Geometry: final body of the model. Coordinates: model frame, mm. Face numbers are marked on the shaded views. A direction names the side the tool comes from. Give positions to 0.01 mm unless a question says otherwise; leave off trailing zeros. Write each loop counter-clockwise with the first axis right and the second up, starting at its lowest first coordinate (ties: lowest second). Pieces come first, ordered by that corner, then holes.
Q1. Cut plane A-A on x = -7.5. Return the cut outline in (y, z) (3 decimals).
Q2. Cut plane C-C on z = -0.5. Return the cut outline in (x, y) (3 decimals).
Q3. Pin query (flat end, axial travel): pin 1 (3 mm diameter, centred on y = -1, z = -4.5, fed in from -X); pin 2 (6 mm diameter, centred on y = -5, z = 3, fed in from -X); pin 3 (2 mm diameter, centred on y = -6.5, z = 7, fed in from +X). Return the tip coordinate at first contact, or that it passes through.
Q4. Line query: L1, parallel to Y at x = 13.25, z = 6.35; L2, parallel to Z at x = 14, y = -19; L3, parallel to Y at x = -13, z = -10.75 (3 decimals). Output: solid intervals per line, ascending.
Q5. Cut plane D-D on x = 14. Return the cut outline in (y, z).
Q6. Cut plane B-B on y = 4.5. Return the cut outline in (x, z), plus the area to 3 significant figures.
Q7. Draft query along X for the marked faces 4, 5 and 6. Return one class per face: pulls with the +X half, pulls with the -X half, needs draft (parallel to the pull), parting line crosses it, or undercut.
Q8. Reachability of the marked faces 1, 2 and 3 from +Z, -Z, +X, -X, +Y, -Y: full face, straight path, thin tool, end or side. Return the list, or none.
```python
from build123d import *

# Parameters (mm, degrees)
SKETCH1_W                      = 38.1
SKETCH1_H                      = 25.4
BOSS_EXTRUDE1_DEPTH            = 12.7
CUT_EXTRUDE2_REACH             = 36.196
SKETCH7_R                      = 3.175
F_6_32_TAPPED_HOLE1_AT_2_COUNT = 2
F_6_32_TAPPED_HOLE1_AT_2_PITCH = 12.7
CUT_EXTRUDE3_DEPTH             = 25.4
SKETCH14_W                     = 28.575
SKETCH14_H                     = 12.7
CUT_EXTRUDE5_DEPTH             = 25.4
FILLET2_R                      = 3.175
FILLET2_OF_MIRROR1_R           = 3.175
FILLET3_R                      = 3.175


with BuildPart() as part:
    # Sketch1 → Boss-Extrude1 (new, symmetric)
    with BuildSketch(Plane.XY):
        Rectangle(SKETCH1_W, SKETCH1_H)
    boss_extrude1 = extrude(amount=BOSS_EXTRUDE1_DEPTH, both=True)

    # Sketch7 → Cut-Extrude2 (cut, up to next)
    with BuildSketch(Plane.XY.offset(12.7), mode=Mode.PRIVATE) as cut_extrude2_sk1:
        with Locations((19.05, -6.35)):
            Circle(SKETCH7_R)
    cut_extrude2_tool1 = extrude(cut_extrude2_sk1.sketch, amount=-CUT_EXTRUDE2_REACH, mode=Mode.PRIVATE) & part.part
    cut_extrude2 = cut_extrude2_tool1.solids().sort_by_distance((19.05, -6.35, 12.7))[0]
    add(cut_extrude2, mode=Mode.SUBTRACT)

    # Sketch11 → #6-32 Tapped Hole1 (revolve, cut)
    with BuildSketch(Plane(origin=(19.05, 6.35, 6.35), x_dir=(0, 0, -1), z_dir=(0, 1, 0))):
        Polygon((0, 0), (0, 8.89), (1.35255, 8.07730597), (1.35255, 0), align=None)
    f_6_32_tapped_hole1 = revolve(axis=Axis((25.4, 6.35, 6.35), (-1, 0, 0)), mode=Mode.SUBTRACT)

    # #6-32 Tapped Hole1 at 2: #6-32 Tapped Hole1 ×2
    with Locations(*[(0, 0, -i * F_6_32_TAPPED_HOLE1_AT_2_PITCH) for i in range(1, F_6_32_TAPPED_HOLE1_AT_2_COUNT)]):
        add(f_6_32_tapped_hole1, mode=Mode.SUBTRACT)

    # Sketch12 → Cut-Extrude3 (cut)
    with BuildSketch(Plane.XY.offset(12.7)):
        with BuildLine():
            Line((-13.335, 9.525), (5.715, 9.525))
            ThreePointArc((5.715, 9.525), (8.89, 6.35), (5.715, 3.175))
            Line((5.715, 3.175), (-13.335, 3.175))
            ThreePointArc((-13.335, 3.175), (-16.51, 6.35), (-13.335, 9.525))
        make_face()
    cut_extrude3 = extrude(amount=-CUT_EXTRUDE3_DEPTH, mode=Mode.SUBTRACT)

    # Sketch14 → Cut-Extrude5 (cut)
    with BuildSketch(Plane.XY.offset(12.7)):
        with Locations((-4.7625, -6.35)):
            Rectangle(SKETCH14_W, SKETCH14_H)
    cut_extrude5 = extrude(amount=-CUT_EXTRUDE5_DEPTH, mode=Mode.SUBTRACT)

    # Fillet2
    fillet2_edges = [part.edges().sort_by_distance(p)[0] for p in [
        (-19.05, 0, 0),
        (9.525, 0, 0),
        (-19.05, 12.7, 0),
    ]]
    fillet(fillet2_edges, radius=FILLET2_R)

    # Mirror1: Boss-Extrude1, Cut-Extrude2, #6-32 Tapped Hole1, Cut-Extrude3, Cut-Extrude5 across plane
    add(boss_extrude1.mirror(Plane.ZX.offset(-6.35)))
    add(cut_extrude2.mirror(Plane.ZX.offset(-6.35)), mode=Mode.SUBTRACT)
    add(f_6_32_tapped_hole1.mirror(Plane.ZX.offset(-6.35)), mode=Mode.SUBTRACT)
    add(cut_extrude3.mirror(Plane.ZX.offset(-6.35)), mode=Mode.SUBTRACT)
    add(cut_extrude5.mirror(Plane.ZX.offset(-6.35)), mode=Mode.SUBTRACT)

    # Mirror1 copy 1 sketch → Mirror1 copy 1 (revolve, cut)
    with BuildSketch(Plane(origin=(19.05, -19.05, -6.35), x_dir=(0, 0, -1), z_dir=(0, -1, 0))):
        Polygon((0, 0), (0, -8.89), (1.35255, -8.07730597), (1.35255, 0), align=None)
    revolve(axis=Axis((25.4, -19.05, -6.35), (1, 0, 0)), mode=Mode.SUBTRACT)

    # Fillet2 of Mirror1
    fillet2_of_mirror1_edges = [part.edges().sort_by_distance(p)[0] for p in [
        (-19.05, -12.7, 0),
        (9.525, -12.7, 0),
        (-19.05, -25.4, 0),
    ]]
    fillet(fillet2_of_mirror1_edges, radius=FILLET2_OF_MIRROR1_R)

    # Fillet3
    fillet3_edges = [part.edges().sort_by_distance(p)[0] for p in [
        (9.525, 0, 0),
    ]]
    fillet(fillet3_edges, radius=FILLET3_R)


solid = part.part
```
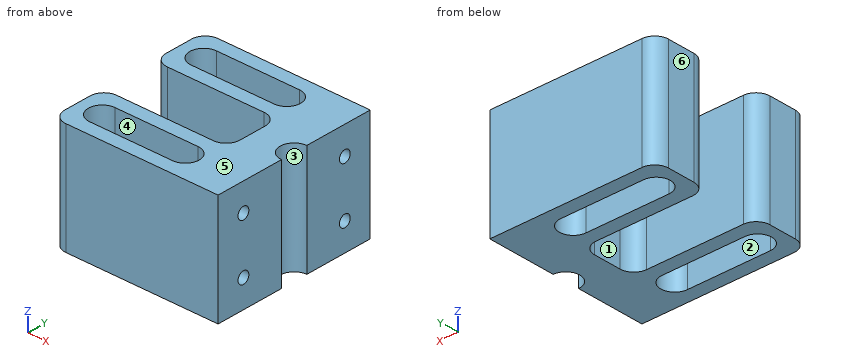
Data:
1. outline: (-25.4, -12.7) - (-22.225, -12.7) - (-22.225, 12.7) - (-25.4, 12.7) - close; (-15.875, -12.7) - (-12.7, -12.7) - (-12.7, 12.7) - (-15.875, 12.7) - close; (0, -12.7) - (3.175, -12.7) - (3.175, 12.7) - (0, 12.7) - close; (9.525, -12.7) - (12.7, -12.7) - (12.7, 12.7) - (9.525, 12.7) - close
2. outline: (-19.05, -22.225) arc R3.175 ccw to (-15.875, -25.4) - (19.05, -25.4) - (19.05, -9.525) arc R3.175 cw to (19.05, -3.175) - (19.05, 12.7) - (-15.875, 12.7) arc R3.175 ccw to (-19.05, 9.525) - (-19.05, 3.175) arc R3.175 ccw to (-15.875, 0) - (6.35, 0) arc R3.175 cw to (9.525, -3.175) - (9.525, -9.525) arc R3.175 cw to (6.35, -12.7) - (-15.875, -12.7) arc R3.175 ccw to (-19.05, -15.875) - close; hole (-13.335, -22.225) - (5.715, -22.225) arc R3.175 ccw to (5.715, -15.875) - (-13.335, -15.875) arc R3.175 ccw to start; hole (-13.335, 3.175) - (5.715, 3.175) arc R3.175 ccw to (5.715, 9.525) - (-13.335, 9.525) arc R3.175 ccw to start
3. pin 1: stops at x = -17.59
3. pin 2: stops at x = 9.3
3. pin 3: stops at x = 16.09
4. L1: y = -25.4 to -20.4, -17.7 to 5, 7.7 to 12.7
4. L2: z = -12.7 to -7.7, -5 to 5, 7.7 to 12.7
4. L3: y = -25.4 to -22.225, -15.875 to -12.7, 0 to 3.175, 9.525 to 12.7
5. outline: (-25.4, -12.7) - (12.7, -12.7) - (12.7, 12.7) - (-25.4, 12.7) - close; hole circle Ø2.71 at (-19.05, -6.35); hole circle Ø2.71 at (-19.05, 6.35); hole circle Ø2.71 at (6.35, -6.35); hole circle Ø2.71 at (6.35, 6.35)
6. outline: (-19.05, -12.7) - (-15.92, -12.7) - (-15.92, 12.7) - (-19.05, 12.7) - close; (8.3, -12.7) - (19.05, -12.7) - (19.05, 12.7) - (8.3, 12.7) - close
6. area: 353 mm2
7. face 4: undercut
7. face 5: needs draft
7. face 6: pulls with the -X half
8. face 1: +Z, -Z, -X
8. face 2: +Z, -Z
8. face 3: +Z, -Z, +X
